Part model, mm, in its own coordinate system. A direction names the side the tool comes from. Coordinates: 2 decimals unless noted, no trailing zeros. Order: outer loops, then holes, each group sorted by start corner. A loop starts at its lowest first (then second) coordinate and runs counter-clockwise, first axis right, second up.
1) Pin check, flat tip, straight feed: pin 1 Ø1 at (y, z) = (8.5, 4) entering from -X. Stop position of the tip, or through.
2) Cut at A-A (x = 62.5). List the corners of the cut face in (y, z).
3) Tool access for faces 5 (the flat face through (0, 15, 4)), 6 (the cylindrical face through (10.59, 20.93, 3.1)), 7 (the flat face through (6.3, 6.9, 2)): list every direction of +Z, -Z, +X, -X, +Y, -Y with a clear straight run to the whole face (end or side of a thin tool).
4) Mould opens along X. For faces 1 (the flat face through (120, 15, 4)), 2 (the flat face through (15, 23, 4)), 3 (the flat face through (59, 15, 7.5)), 4 (the flat face through (6.3, 21.9, 2)) say: +X half, -X half, draft (parallel to the pull), parting line (faces both ways), or undercut.
5) Wall check: L1, parallel to Y at x = 86, z = 6; L2, parallel to X at y = 25, z = 4.5; L3, parallel to Y at x = 112.5, z = 7. Give the ranges that are in metal, low to high.
6) Cut at D-D (z = 3.75). Give the number of separate pieces and of enclosed holes in the cut face, and give its area (3 significant figures).
7) Cut at C-C (x = 10). List the corners of the cut face in (y, z).
8) Cut at B-B (y = 7.5). List the corners of the cut face in (x, z), and give its area (3 significant figures).
```python
from build123d import *

# Parameters (mm, degrees)
SKETCH_W     = 120
SKETCH_H     = 30
SKETCH_W_2   = 2.3
SKETCH_H_2   = 5.55
PAD_DEPTH    = 7.5
SKETCH001_R  = 1.7
POCKET_DEPTH = 15


with BuildPart() as part:
    # Sketch → Pad (new body)
    with BuildSketch(Plane.XY):
        with Locations((60, 15)):
            Rectangle(SKETCH_W, SKETCH_H)
        with Locations((5.15, 22.525)):
            Rectangle(SKETCH_W_2, SKETCH_H_2, mode=Mode.SUBTRACT)
        with Locations((5.15, 7.525)):
            Rectangle(SKETCH_W_2, SKETCH_H_2, mode=Mode.SUBTRACT)
        with BuildLine():
            ThreePointArc((32, 24.2), (30.3, 22.5), (32, 20.8))
            Line((32, 20.8), (112, 20.8))
            ThreePointArc((112, 20.8), (113.7, 22.5), (112, 24.2))
            Line((32, 24.2), (112, 24.2))
        make_face(mode=Mode.SUBTRACT)
        with BuildLine():
            ThreePointArc((32, 9.2), (30.3, 7.5), (32, 5.8))
            Line((32, 5.8), (112, 5.8))
            ThreePointArc((112, 5.8), (113.7, 7.5), (112, 9.2))
            Line((32, 9.2), (112, 9.2))
        make_face(mode=Mode.SUBTRACT)
    extrude(amount=PAD_DEPTH)

    # Sketch001 (on Face4 of Pad) → Pocket (cut)
    with BuildSketch(Plane(origin=(0, 0, 0), x_dir=(0, -1, 0), z_dir=(-1, 0, 0))):
        with Locations((-22.5, 3.75)):
            Circle(SKETCH001_R)
        with Locations((-7.5, 3.75)):
            Circle(SKETCH001_R)
    extrude(amount=-POCKET_DEPTH, mode=Mode.SUBTRACT)


solid = part.part
```
Geometry check:
1. pin 1: stops at x = 15
2. outline: (0, 0) - (5.8, 0) - (5.8, 7.5) - (0, 7.5) - close; (9.2, 0) - (20.8, 0) - (20.8, 7.5) - (9.2, 7.5) - close; (24.2, 0) - (30, 0) - (30, 7.5) - (24.2, 7.5) - close
3. face 5: +Z, -Z, -X, +Y, -Y
3. face 6: -X
3. face 7: +Z, -Z
4. face 1: +X half
4. face 2: -X half
4. face 3: draft
4. face 4: undercut
5. L1: y = 0 to 5.8, 9.2 to 20.8, 24.2 to 30
5. L2: x = 0 to 4, 6.3 to 120
5. L3: y = 0 to 5.88, 9.12 to 20.88, 24.12 to 30
6. separate pieces: 1
6. enclosed holes: 2
6. area: 2,930 mm2
7. outline: (0, 0) - (30, 0) - (30, 7.5) - (0, 7.5) - close; hole circle Ø3.4 at (7.5, 3.75); hole circle Ø3.4 at (22.5, 3.75)
8. outline: (0, 0) - (4, 0) - (4, 2.05) - (0, 2.05) - close; (0, 5.45) - (4, 5.45) - (4, 7.5) - (0, 7.5) - close; (6.3, 0) - (30.3, 0) - (30.3, 7.5) - (6.3, 7.5) - (6.3, 5.45) - (15, 5.45) - (15, 2.05) - (6.3, 2.05) - close; (113.7, 0) - (120, 0) - (120, 7.5) - (113.7, 7.5) - close
8. area: 214 mm2
